The model under review builds one solid part; all positions refer to its coordinate system, in mm. Face numbers are marked on the shaded views. Coordinates: 2 decimals unless noted, no trailing zeros. Loops run counter-clockwise (first coordinate to the right, second up) from the corner with the lowest first, then second, coordinate; pieces in that order, holes last. Notation, with made-up numbers: M 26.25,2 L 38.25,2 A24 ccw 38.25,13 Z; hole C 53.25,9.5 d3. An arc over 180 degrees is marked long. Return JSON: item names as keys, results as strings.
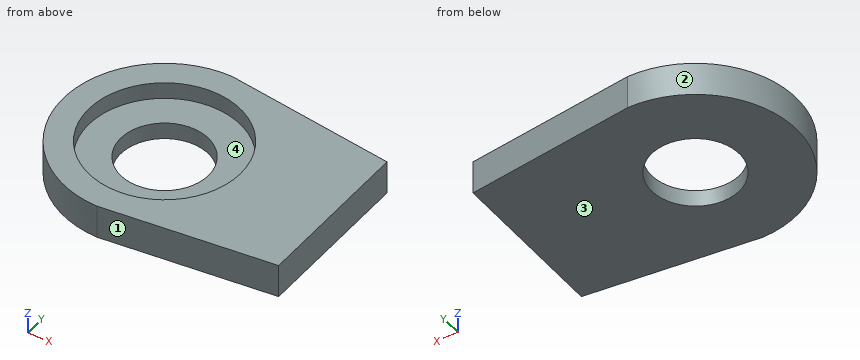
```python
from build123d import *

# Parameters (mm, degrees)
BOSS_EXTRUDE1_DEPTH = 2
SKETCH5_R           = 2.6
CUT_EXTRUDE1_DEPTH  = 2
SKETCH6_R           = 4.5
CUT_EXTRUDE2_DEPTH  = 1


with BuildPart() as part:
    # Sketch2 → Boss-Extrude1 (new body)
    with BuildSketch(Plane.XY):
        with BuildLine():
            Line((10, -4.8), (10, 4.8))
            Line((10, 4.8), (0, 6))
            ThreePointArc((0, 6), (-6, 0), (0, -6))
            Line((0, -6), (10, -4.8))
        make_face()
    extrude(amount=BOSS_EXTRUDE1_DEPTH)

    # Sketch5 → Cut-Extrude1 (cut)
    with BuildSketch(Plane.XY.offset(2)):
        Circle(SKETCH5_R)
    extrude(amount=-CUT_EXTRUDE1_DEPTH, mode=Mode.SUBTRACT)

    # Sketch6 → Cut-Extrude2 (cut)
    with BuildSketch(Plane.XY.offset(2)):
        Circle(SKETCH6_R)
    extrude(amount=-CUT_EXTRUDE2_DEPTH, mode=Mode.SUBTRACT)


solid = part.part
```
1. Add section D-D on x = -4.25. Give the boundary of the cut face in (y, z).
Check values:
{"outline": "M -4.24,0 L 4.24,0 L 4.24,2 L 1.48,2 L 1.48,1 L -1.48,1 L -1.48,2 L -4.24,2 Z"}
2. Add section A-A on y = 0. Give the boundary of the cut face in (x, z), plus the area to 3 significant figures.
Check values:
{"outline": "M -6,0 L -2.6,0 L -2.6,1 L -4.5,1 L -4.5,2 L -6,2 Z; M 2.6,0 L 10,0 L 10,2 L 4.5,2 L 4.5,1 L 2.6,1 Z", "area": "17.8 mm²"}
3. Add section B-B on z = 1.2. Give the boundary of the cut face in (x, y).
Check values:
{"outline": "M 0,-6 L 10,-4.8 L 10,4.8 L 0,6 A6 ccw Z; hole C 0,0 d9"}
4. The part is to be moulded in two halves that separate along X. For the marked faces 1, 2, 3 and 4, say which applies: released by +X, released by -X, zero draft, split by the parting line, or undercut.
Check values:
{"face 1": "released by +X", "face 2": "released by -X", "face 3": "zero draft", "face 4": "undercut"}
5. To check wall thickness, follow line 1 (Z direction, x = 0.75, y = -2.75); line 2 (X direction, y = -3, z = 1.85); line 3 (X direction, y = 1.75, z = 0.9). State the ranges of each line that lie inside material, in increasing order.
Check values:
{"line 1": "0 to 1", "line 2": "-5.2 to -3.35, 3.35 to 10", "line 3": "-5.74 to -1.92, 1.92 to 10"}
6. Add section C-C on x = -1.5. Give the boundary of the cut face in (y, z), plus the area to 3 significant figures.
Check values:
{"outline": "M -5.81,0 L -2.12,0 L -2.12,1 L -4.24,1 L -4.24,2 L -5.81,2 Z; M 2.12,0 L 5.81,0 L 5.81,2 L 4.24,2 L 4.24,1 L 2.12,1 Z", "area": "10.5 mm²"}
7. Insertion check: pin 1 Ø1 at (x, y) = (4, -4.5) entering from -Z; pin 2 Ø3 at (x, y) = (0, 0) entering from +Z. Each pin has a flat end and moves straight along its axis. Give the tip position at first contact, or say it passes through.
Check values:
{"pin 1": "z = 0", "pin 2": "through"}
